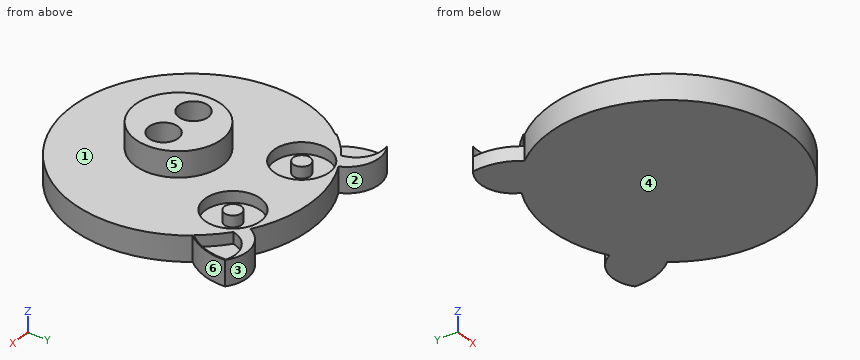
from build123d import *

# Parameters (mm, degrees)
F1_DEPTH = 6.35
F2_R     = 10.8590085074
F2_R_2   = 3.6802492117
F3_DEPTH = 6.35
F4_R     = 6.9693581069
F4_R_2   = 2.1365687552
F5_DEPTH = 2.8448


with BuildPart() as f1:
    # F0 (on Top) → F1 (new body)
    with BuildSketch(Plane.XY):
        with BuildLine():
            ThreePointArc((22.1884083003, 32.5379781425), (15.3640692537, 34.0499493944), (9.9405326157, 29.6405377755))
            ThreePointArc((9.9405326157, 29.6405377755), (-4.6095652506, 33.4153325113), (-19.1596631168, 29.6405377755))
            ThreePointArc((-19.1596631168, 29.6405377755), (-24.5831997549, 34.0499493944), (-31.4075388014, 32.5379781425))
            ThreePointArc((-31.4075388014, 32.5379781425), (-30.8582548555, 26.9031615507), (-28.2005693571, 21.9042037926))
            ThreePointArc((-28.2005693571, 21.9042037926), (-4.6095652506, -26.4433986324), (18.981438856, 21.9042037926))
            ThreePointArc((18.981438856, 21.9042037926), (21.6391243544, 26.9031615507), (22.1884083003, 32.5379781425))
        make_face()
    extrude(amount=F1_DEPTH)

    # F2 (on face) → F3 (join)
    with BuildSketch(Plane.XY.offset(6.35)):
        with Locations((-4.8612458631, 0.0010582291)):
            Circle(F2_R)
        with Locations((-9.8135089502, 0.0010582291)):
            Circle(F2_R_2, mode=Mode.SUBTRACT)
        with Locations((0.0910172239, 0.0010582291)):
            Circle(F2_R_2, mode=Mode.SUBTRACT)
    extrude(amount=F3_DEPTH)

    # F4 (on face) → F5 (cut)
    with BuildSketch(Plane.XY.offset(6.35)):
        with BuildLine():
            ThreePointArc((-31.4075388014, 32.5379781425), (-30.8945224978, 27.0253518282), (-28.359989317, 22.103118985))
            ThreePointArc((-28.359989317, 22.103118985), (-25.7072477965, 25.0367408797), (-22.6908403268, 27.5949552906))
            ThreePointArc((-22.6908403268, 27.5949552906), (-25.7360645395, 32.0302919162), (-31.0613331918, 32.7965263897))
            ThreePointArc((-31.0613331918, 32.7965263897), (-31.2361754941, 32.6695815173), (-31.4075388014, 32.5379781425))
        make_face()
        with Locations((-16.254756134, 22.5346526879)):
            Circle(F4_R)
        with Locations((-16.254756134, 22.5346526879)):
            Circle(F4_R_2, mode=Mode.SUBTRACT)
        with Locations((6.4890854992, 22.5346526879)):
            Circle(F4_R)
        with Locations((6.4890854992, 22.5346526879)):
            Circle(F4_R_2, mode=Mode.SUBTRACT)
        with BuildLine():
            ThreePointArc((12.925169692, 27.5949552906), (16.007657655, 24.9725297062), (18.7081687892, 21.9582159201))
            ThreePointArc((18.7081687892, 21.9582159201), (21.3658542875, 26.9571736782), (21.9151382335, 32.59199027))
            ThreePointArc((21.9151382335, 32.59199027), (16.251635807, 32.1957077064), (12.925169692, 27.5949552906))
        make_face()
    extrude(amount=-F5_DEPTH, mode=Mode.SUBTRACT)


solid = f1.part
Input: part model. Units: mm. Frame: model coordinates. Face numbers are marked on the shaded views. A direction names the side the tool comes from. Coordinates: 2 decimals unless noted, no trailing zeros. Write each loop counter-clockwise with the first axis right and the second up, starting at its lowest first coordinate (ties: lowest second). Pieces come first, ordered by that corner, then holes. Notation, with made-up numbers: M 60,43.5 L 106,43.5 A35 cw 106,81.5 Z; hole C -6.5,65 d7. An arc over 180 degrees is marked long. Answer as a JSON object with one key per item and string values. Group by question number.
(1) Section B-B on y = 9. Output: boundary loops of the cut face in (x, z), plus the area to 3 significant figures.
(2) Ray query, line 1 along X through (y, z) = (23.5, 6.25); line 2 along Z through (x, y) = (-2.5, -1.5); line 3 along Z through (x, y) = (21, 29.5). Return the intervals inside material, ascending. Write a range as [from, to].
(3) Section A-A on z = 4.75. Output: boundary loops of the cut face in (x, y), plus the area to 3 significant figures.
(4) Set-up query: the marked faces 1 and 2. Return all of +Z, -Z, +X, -X, +Y, -Y with unobstructed straight access to the full face (end or side cutting, diameter ignored); none if empty.
(5) Section D-D on z = 9.25. Output: boundary loops of the cut face in (x, y).
(6) Section C-C on x = -5. Output: boundary loops of the cut face in (y, z).
(7) Mould query, pull axis X, two halves, no side actions, for the marked faces 3, 4, 5 and 6. Classes: pulls with the +X half, pulls with the -X half, needs draft (parallel to the pull), parting line crosses it, or undercut.
(8) Contact query for flat-ended pins moving along their axis: P1, Ø11, axis at x = 5, y = 21, coming from the +Z side; P2, Ø6, axis at x = 14.5, z = 6.5, coming from the -Y side; P3, Ø4, axis at x = -20.5, z = 7, coming from the +Y side. Output: stop coordinate, or through.
Result set:
{
 "1": {"outline": "M -34.03,0 L 24.81,0 L 24.81,6.35 L 1.22,6.35 L 1.22,12.7 L -10.94,12.7 L -10.94,6.35 L -34.03,6.35 Z", "area": "451 mm2"},
 "2": {"line 1": "x = [-27.18, -23.16], [-18.16, -14.35], [-9.35, -0.41], [4.58, 8.4], [13.39, 17.42], [19.81, 20.11]", "line 2": "z = [0, 6.35]", "line 3": "z = [0, 3.51]"},
 "3": {"outline": "M -31.06,32.8 A6.7 cw -22.69,27.59 A29.93 ccw -28.36,22.1 A14.55 ccw -28.2,21.9 A29.93 ccw long 18.98,21.9 A14.55 ccw 22.19,32.54 A8.03 ccw 9.94,29.64 A29.93 ccw -19.16,29.64 A8.03 ccw Z; C -16.25,22.53 d4.27; C 6.49,22.53 d4.27; hole C -16.25,22.53 d13.94; hole C 6.49,22.53 d13.94; hole M 12.93,27.59 A29.93 cw 18.71,21.96 A14.55 ccw 21.92,32.59 A6.7 ccw Z", "area": "2,590 mm2"},
 "4": {"face 1": "+Z", "face 2": "+Z, -Z, +Y"},
 "5": {"outline": "C -4.86,0 d21.72; hole C -9.81,0 d7.36; hole C 0.09,0 d7.36"},
 "6": {"outline": "M -26.44,0 L 33.41,0 L 33.41,6.35 L 10.86,6.35 L 10.86,12.7 L -10.86,12.7 L -10.86,6.35 L -26.44,6.35 Z"},
 "7": {"face 3": "undercut", "face 4": "needs draft", "face 5": "parting line crosses it", "face 6": "pulls with the +X half"},
 "8": {"P1": "stops at z = 6.35", "P2": "stops at y = -21.74", "P3": "stops at y = 33.18"}
}
